The listing builds one solid part. Answer for the finished solid, in the listing's coordinates (mm). A direction names the side the tool comes from. Round coordinates to 2 decimals unless told otherwise and drop trailing zeros. Loops run counter-clockwise (first coordinate to the right, second up) from the corner with the lowest first, then second, coordinate; pieces in that order, holes last. Notation, with made-up numbers: M -36,76 L 5,76 A24 ccw 5,106 Z; hole C -29,75 d2. An arc over 180 degrees is marked long. Answer as a JSON object with one key per item and string values.
```python
from build123d import *

# Parameters (mm, degrees)
SKETCH1_W                      = 80
SKETCH1_H                      = 78
BOSS_EXTRUDE1_DEPTH            = 8.4
SKETCH4_W                      = 5.08
SKETCH4_H                      = 1.905
CUT_EXTRUDE1_DEPTH             = 9.4
LPATTERN1_COUNT                = 2
LPATTERN1_PITCH                = 19
LPATTERN1_COUNT_DIR2           = 2
LPATTERN1_PITCH_DIR2           = 48
SKETCH5_W                      = 5.08
SKETCH5_H                      = 1.905
CUT_EXTRUDE2_DEPTH             = 8.4
LPATTERN2_COUNT                = 2
LPATTERN2_PITCH                = 19
CUT_EXTRUDE3_DEPTH             = 9.4
CUT_EXTRUDE4_DEPTH             = 2.138
SKETCH9_R                      = 1.5875
CUT_EXTRUDE5_DEPTH             = 9.4
SKETCH11_W                     = 80
SKETCH11_H                     = 8.4
BOSS_EXTRUDE3_DEPTH            = 10
F_2_5_2_5_DIAMETER_HOLE1_D     = 2.5
F_2_5_2_5_DIAMETER_HOLE1_DEPTH = 10
SKETCH14_W                     = 9
SKETCH14_H                     = 8.4
SKETCH14_W_2                   = 7
BOSS_EXTRUDE4_DEPTH            = 15
SKETCH16_R                     = 2
CUT_EXTRUDE6_DEPTH             = 45.4
FILLET1_R                      = 4


with BuildPart() as part:
    # Sketch1 → Boss-Extrude1 (new body)
    with BuildSketch(Plane.XY):
        with Locations((40, 39)):
            Rectangle(SKETCH1_W, SKETCH1_H)
    extrude(amount=BOSS_EXTRUDE1_DEPTH)

    # Sketch2 → Cut-Revolve1 (revolve, cut)
    with BuildSketch(Plane.XY.offset(8.4)):
        Polygon((0, 70.5), (0, 64), (9.541087991, 64), (23.495378694, 64), (54.462434776, 64), (68.225570813, 64), (80, 64), (80, 70.5), (76, 70.5), (76, 71.5), (52, 71.5), (52, 70.5), (28, 70.5), (28, 71.5), (4, 71.5), (4, 70.5), align=None)
    revolve(axis=Axis((0, 64, 8.4), (1, 0, 0)), mode=Mode.SUBTRACT)

    # Sketch3 → Cut-Revolve2 (revolve, cut)
    with BuildSketch(Plane.XY.offset(8.4)):
        Polygon((0, 20.5), (0, 14), (25.709253363, 14), (47.957380272, 14), (80, 14), (80, 20.5), (52, 20.5), (52, 21.5), (28, 21.5), (28, 20.5), align=None)
    revolve(axis=Axis((0, 14, 8.4), (1, 0, 0)), mode=Mode.SUBTRACT)

    # Sketch4 → Cut-Extrude1 (cut, through all)
    with BuildSketch(Plane.XY.offset(8.4)):
        with Locations((8.54, 73.4525)):
            Rectangle(SKETCH4_W, SKETCH4_H)
        with Locations((23.46, 73.4525)):
            Rectangle(SKETCH4_W, SKETCH4_H)
    cut_extrude1 = extrude(amount=-CUT_EXTRUDE1_DEPTH, mode=Mode.SUBTRACT)

    # LPattern1: Cut-Extrude1 2 × 2
    with Locations(*[(j * LPATTERN1_PITCH_DIR2, -i * LPATTERN1_PITCH, 0) for i in range(LPATTERN1_COUNT) for j in range(LPATTERN1_COUNT_DIR2) if (i, j) != (0, 0)]):
        add(cut_extrude1, mode=Mode.SUBTRACT)

    # Sketch5 → Cut-Extrude2 (cut)
    with BuildSketch(Plane.XY.offset(8.4)):
        with Locations((32.54, 23.5525)):
            Rectangle(SKETCH5_W, SKETCH5_H)
        with Locations((47.46, 23.5525)):
            Rectangle(SKETCH5_W, SKETCH5_H)
    cut_extrude2 = extrude(amount=-CUT_EXTRUDE2_DEPTH, mode=Mode.SUBTRACT)

    # LPattern2: Cut-Extrude2 ×2
    with Locations(*[(0, -i * LPATTERN2_PITCH, 0) for i in range(1, LPATTERN2_COUNT)]):
        add(cut_extrude2, mode=Mode.SUBTRACT)

    # Sketch6 → Cut-Extrude3 (cut, through all)
    with BuildSketch(Plane.XY.offset(8.4)):
        with BuildLine():
            ThreePointArc((62.017883983, 42.650499467), (61.02396367, 42.911979229), (60, 43))
            ThreePointArc((60, 43), (54, 37), (60, 31))
            ThreePointArc((60, 31), (61.02396367, 31.088020771), (62.017883983, 31.349500533))
            Line((62.017883983, 31.349500533), (64, 31))
            Line((64, 31), (80, 31))
            Line((80, 31), (80, 43))
            Line((80, 43), (64, 43))
            Line((64, 43), (62.017883983, 42.650499467))
        make_face()
    extrude(amount=-CUT_EXTRUDE3_DEPTH, mode=Mode.SUBTRACT)

    # Sketch8 → Cut-Extrude4 (cut)
    with BuildSketch(Plane.XY.offset(8.4)):
        with BuildLine():
            Line((80, 45), (80, 29))
            Line((80, 29), (63.825022673, 29))
            Line((63.825022673, 29), (62.152264354, 29.294952424))
            ThreePointArc((62.152264354, 29.294952424), (52, 37), (62.152264354, 44.705047576))
            Line((62.152264354, 44.705047576), (63.825022673, 45))
            Line((63.825022673, 45), (80, 45))
        make_face()
    extrude(amount=-CUT_EXTRUDE4_DEPTH, mode=Mode.SUBTRACT)

    # Sketch9 → Cut-Extrude5 (cut, through all)
    with BuildSketch(Plane.XY.offset(8.4)):
        with Locations((10, 35)):
            Circle(SKETCH9_R)
        with Locations((28, 35)):
            Circle(SKETCH9_R)
    extrude(amount=-CUT_EXTRUDE5_DEPTH, mode=Mode.SUBTRACT)

    # Sketch11 → Boss-Extrude3 (add)
    with BuildSketch(Plane(origin=(0, 0, 0), x_dir=(-1, 0, 0), z_dir=(0, -1, 0))):
        with Locations((-40, -4.2)):
            Rectangle(SKETCH11_W, SKETCH11_H)
    extrude(amount=BOSS_EXTRUDE3_DEPTH)

    # Ø2.5 (2.5) Diameter Hole1
    with Locations(Plane.XY.offset(8.4)):
        with Locations((40, -5.5)):
            Hole(F_2_5_2_5_DIAMETER_HOLE1_D / 2, depth=F_2_5_2_5_DIAMETER_HOLE1_DEPTH)

    # Sketch14 → Boss-Extrude4 (add)
    with BuildSketch(Plane(origin=(0, 78, 0), x_dir=(1, 0, 0), z_dir=(0, 1, 0))):
        with Locations((60, -4.2)):
            Rectangle(SKETCH14_W, SKETCH14_H)
        with Locations((76.5, -4.2)):
            Rectangle(SKETCH14_W_2, SKETCH14_H)
        with Locations((43.5, -4.2)):
            Rectangle(SKETCH14_W_2, SKETCH14_H)
    extrude(amount=BOSS_EXTRUDE4_DEPTH)

    # Sketch16 → Cut-Extrude6 (cut)
    with BuildSketch(Plane.ZY.offset(-40)):
        with Locations((4.2, 88)):
            Circle(SKETCH16_R)
    extrude(amount=-CUT_EXTRUDE6_DEPTH, mode=Mode.SUBTRACT)

    # Fillet1
    fillet1_edges = [part.edges().sort_by_distance(p)[0] for p in [
        (76.5, 93, 8.4),
        (76.5, 93, 0),
        (60, 93, 8.4),
        (60, 93, 0),
        (43.5, 93, 8.4),
        (43.5, 93, 0),
    ]]
    fillet(fillet1_edges, radius=FILLET1_R)


solid = part.part
```
Item 1: The part is cut by section C-C (x = 48.5). Give the vertices of the cut face in (y, z) (3 decimals).
Values follow:
{"outline": "M -10,0 L 3.6,0 L 3.6,8.4 L -10,8.4 Z; M 5.505,0 L 22.6,0 L 22.6,8.4 L 21.5,8.4 A7.5 cw 6.5,8.4 L 5.505,8.4 Z; M 24.505,0 L 78,0 L 78,8.4 L 70.5,8.4 A6.5 cw 57.5,8.4 L 24.505,8.4 Z"}
Item 2: Determine the mould class of faces 1 (the face through (76.549, 91.859, 1.203)), 2 (the face through (28, 63.5, 1.6)) for opening direction X: released by +X, released by -X, zero draft, split by the parting line, or undercut.
Values follow:
{"face 1": "zero draft", "face 2": "undercut"}
Item 3: The part is cut by section D-D (y = 14). Give the vertices of the cut face in (x, z), then the cut area to 3 significant figures.
Values follow:
{"outline": "M 0,0 L 80,0 L 80,1.9 L 52,1.9 L 52,0.9 L 28,0.9 L 28,1.9 L 0,1.9 Z", "area": "128 mm^2"}
Item 4: Straight lines are drawn through the part: line 1 (Y direction, x = 22.5, z = 0.75) (3 decimals); line 2 (X direction, y = 82.5, z = 3.5); line 3 (Y direction, x = 66, z = 0.75). For each, find the intervals that lie inside material, in ascending order.
Values follow:
{"line 1": "-10 to 53.5, 55.405 to 72.5, 74.405 to 78", "line 2": "40 to 47, 55.5 to 64.5, 73 to 80", "line 3": "-10 to 31, 43 to 78"}
Item 5: The part is cut by section A-A (x = 10). Give the vertices of the cut face in (y, z) (1 decimal), then the cut area to 3 significant figures.
Values follow:
{"outline": "M -10,0 L 33.4,0 L 33.4,8.4 L 20.5,8.4 A6.5 cw 7.5,8.4 L -10,8.4 Z; M 36.6,0 L 53.5,0 L 53.5,8.4 L 36.6,8.4 Z; M 55.4,0 L 72.5,0 L 72.5,8.4 L 71.5,8.4 A7.5 cw 56.5,8.4 L 55.4,8.4 Z; M 74.4,0 L 78,0 L 78,8.4 L 74.4,8.4 Z", "area": "526 mm^2"}
Item 6: Flat-ended cylindrical pins translate along their axes: P1, Ø2.5, axis at x = 48, z = 6, coming from the +Y side; P2, Ø5, axis at y = 88, z = 4.2, coming from the -X side. Find the tip coordinate at first contact, or state that the pin passes through.
Values follow:
{"P1": "y = 92.91", "P2": "x = 40"}
Item 7: Which of the six approach directions +Z, -Z, +X, -X, +Y, -Y give full straight-line access (tool end or side, diameter ignored) to faces 3 (the face through (20, 78, 4)), 4 (the face through (65.8, 13.9, 1.9)), 5 (the face through (69, 78, 4)), 6 (the face through (47, 3.6, 4))?
Values follow:
{"face 3": "+Z, -Z, -X, +Y", "face 4": "+Z, +X, -X", "face 5": "+Z, -Z, +Y", "face 6": "+Z, -Z"}
Item 8: The part is cut by section B-B (y = 81). Give the vertices of the cut face in (x, z).
Values follow:
{"outline": "M 40,0 L 47,0 L 47,8.4 L 40,8.4 Z; M 55.5,0 L 64.5,0 L 64.5,8.4 L 55.5,8.4 Z; M 73,0 L 80,0 L 80,8.4 L 73,8.4 Z"}
